Source: three-view drawing plus pictorial views. Frame: mm from the lowest corner of the part. A direction names the side the tool comes from. Give positions to 0.01 mm unless a question says otherwise; leave off trailing zeros. Loops run counter-clockwise (first coordinate to the right, second up) from the corner with the lowest first, then second, coordinate; pieces in that order, holes last. Notation, with made-up numbers: (46, 54.25) - (91, 54.25) arc R22 ccw to (91, 84.25) - close; hole circle Ø6 at (16.5, 55.5). An arc over 180 degrees is marked (long way). Answer as a JSON object with one key per item and string values. Group by question number.
(1) Material intervals for L1, parallel to Y at x = 19, z = 1.75; L2, parallel to X at y = 12.5, z = 1.45; L3, parallel to Y at x = 5, z = 4.65, sorted ascending.
(2) Pin query (flat end, axial travel): P1, Ø2, axis at x = 6, y = 7, coming from the +Z side. Return the tip coordinate at first contact, or that it passes through.
(3) Section query A-A (x = 32.5). Return loops of the section in (y, z).
(4) Mould query, pull axis Y, two halves, no side actions, for the marked faces 3, 4, 5 and 6. Classes: +Y half, -Y half, draft (parallel to the pull), parting line (faces both ways), or undercut.
(5) Section query D-D (x = 25.5). Return loops of the section in (y, z).
(6) Section query B-B (z = 4.05). Return loops of the section in (x, y).
(7) Section query C-C (y = 14). Return loops of the section in (x, z).
(8) Access query for the marked faces 1 and 2. Directions: +Z, -Z, +X, -X, +Y, -Y. A direction counts if a zero-diameter tool reaches every point of the face in a straight line with its end or side. Return the directions, or none.
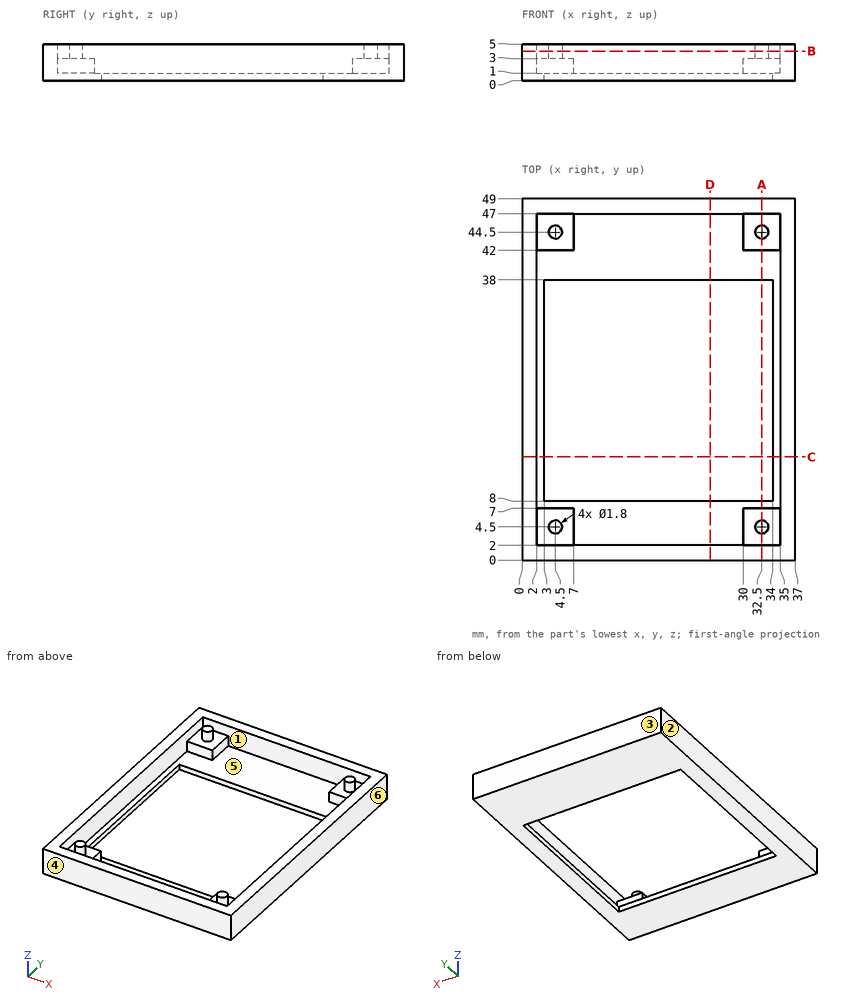
Recorded:
{
 "1": {"L1": "y = 0 to 2, 47 to 49", "L2": "x = 0 to 2, 35 to 37", "L3": "y = 0 to 2, 3.75 to 5.25, 43.75 to 45.25, 47 to 49"},
 "2": {"P1": "stops at z = 3"},
 "3": {"outline": "(0, 0) - (8, 0) - (8, 1) - (7, 1) - (7, 3) - (5.4, 3) - (5.4, 5) - (3.6, 5) - (3.6, 3) - (2, 3) - (2, 5) - (0, 5) - close; (38, 0) - (49, 0) - (49, 5) - (47, 5) - (47, 3) - (45.4, 3) - (45.4, 5) - (43.6, 5) - (43.6, 3) - (42, 3) - (42, 1) - (38, 1) - close"},
 "4": {"face 3": "+Y half", "face 4": "-Y half", "face 5": "undercut", "face 6": "draft"},
 "5": {"outline": "(0, 0) - (8, 0) - (8, 1) - (2, 1) - (2, 5) - (0, 5) - close; (38, 0) - (49, 0) - (49, 5) - (47, 5) - (47, 1) - (38, 1) - close"},
 "6": {"outline": "(0, 0) - (37, 0) - (37, 49) - (0, 49) - close; circle Ø1.8 at (4.5, 4.5); circle Ø1.8 at (4.5, 44.5); circle Ø1.8 at (32.5, 4.5); circle Ø1.8 at (32.5, 44.5); hole (2, 2) - (35, 2) - (35, 47) - (2, 47) - close"},
 "7": {"outline": "(0, 0) - (3, 0) - (3, 1) - (2, 1) - (2, 5) - (0, 5) - close; (34, 0) - (37, 0) - (37, 5) - (35, 5) - (35, 1) - (34, 1) - close"},
 "8": {"face 1": "+Z", "face 2": "+Z, -Z, -X, +Y, -Y"}
}
